from build123d import *

# Parameters (mm, degrees)
SKETCH1_W           = 20
SKETCH1_H           = 405
BOSS_EXTRUDE1_DEPTH = 5
CUT_EXTRUDE1_REACH  = 409.6
SKETCH3_R           = 16.7


with BuildPart() as part:
    # Sketch1 → Revolve1 (revolve)
    with BuildSketch(Plane.XY, mode=Mode.PRIVATE) as revolve1_sk:
        with Locations((10, 202.5)):
            Rectangle(SKETCH1_W, SKETCH1_H)
    revolve(revolve1_sk.sketch.rotate(Axis((0, 405, 0), (0, -1, 0)), 180), axis=Axis((0, 405, 0), (0, -1, 0)))

    # Sketch2 → Boss-Extrude1 (add)
    with BuildSketch(Plane(origin=(0, 405, 0), x_dir=(1, 0, 0), z_dir=(0, 1, 0))):
        with BuildLine():
            Line((-20.5, -32.5), (20.5, -32.5))
            ThreePointArc((20.5, -32.5), (28.985281374, -28.985281374), (32.5, -20.5))
            Line((32.5, -20.5), (32.5, 20.5))
            ThreePointArc((32.5, 20.5), (28.985281374, 28.985281374), (20.5, 32.5))
            Line((20.5, 32.5), (-20.5, 32.5))
            ThreePointArc((-20.5, 32.5), (-28.985281374, 28.985281374), (-32.5, 20.5))
            Line((-32.5, 20.5), (-32.5, -20.5))
            ThreePointArc((-32.5, -20.5), (-28.985281374, -28.985281374), (-20.5, -32.5))
        make_face()
    extrude(amount=-BOSS_EXTRUDE1_DEPTH)

    # Sketch3 → Cut-Extrude1 (cut, up to next)
    with BuildSketch(Plane.XZ, mode=Mode.PRIVATE) as cut_extrude1_sk1:
        Circle(SKETCH3_R)
    cut_extrude1_tool1 = extrude(cut_extrude1_sk1.sketch, amount=-CUT_EXTRUDE1_REACH, mode=Mode.PRIVATE) & part.part
    add(cut_extrude1_tool1.solids().sort_by_distance((0, 0, 0))[0], mode=Mode.SUBTRACT)


solid = part.part
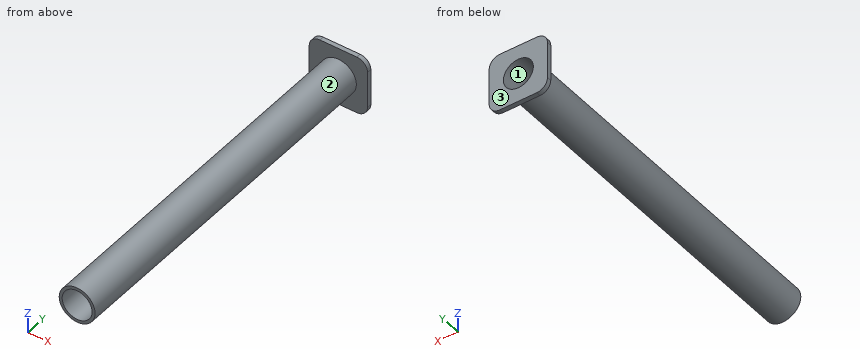
Could you check a few things on this model? Use its own coordinates, in mm. Face numbers are marked on the shaded views. Round coordinates to 2 decimals unless told otherwise and drop trailing zeros. Order: outer loops, then holes, each group sorted by start corner. A loop starts at its lowest first (then second) coordinate and runs counter-clockwise, first axis right, second up.
Q1. Thinking about a two-plate mould opening in Z: for the marked faces 1, 2 and 3, which applies, released by +Z, released by -Z, zero draft, split by the parting line, or undercut?
Geometry says:
face 1: undercut
face 2: split by the parting line
face 3: zero draft
Q2. Imagine slicing it at C-C, the plane y = 134. List the corners of the cut face in (x, z) for me.
Geometry says:
outline: circle Ø40 at (0, 0); hole circle Ø33.4 at (0, 0)
Q3. I'm going to push flat-ended pins straight in: P1, Ø1.5, axis at y = 60, z = 2.5, coming from the -X side; P2, Ø3, axis at x = 15.5, y = 279.5, coming from the -Z side; P3, Ø5, axis at y = 96.5, z = 11, coming from the +X side; P4, Ø20, axis at x = 0, z = 0, coming from the -Y side. Where does each tip first touch, or does it pass through?
Geometry says:
P1: stops at x = -19.92
P2: stops at z = -14.28
P3: stops at x = 18.1
P4: passes through
Q4. Imagine slicing it at A-A, the plane z = 0. List the corners of the cut face in (x, y) for me.
Geometry says:
outline: (-32.5, 400) - (-20, 400) - (-20, 0) - (-16.7, 0) - (-16.7, 405) - (-32.5, 405) - close; (16.7, 0) - (20, 0) - (20, 400) - (32.5, 400) - (32.5, 405) - (16.7, 405) - close
Q5. Imagine slicing it at B-B, the plane x = 0. List the corners of the cut face in (y, z) for me, then the cut area to 3 significant figures.
Geometry says:
outline: (0, -20) - (400, -20) - (400, -32.5) - (405, -32.5) - (405, -16.7) - (0, -16.7) - close; (0, 16.7) - (405, 16.7) - (405, 32.5) - (400, 32.5) - (400, 20) - (0, 20) - close
area: 2,800 mm2
Q6. Please list where these lines run through material, in increasing order: probe 1 along Z at (x, y) = (0, 228); probe 2 along Y at (x, z) = (-10, 26.5); probe 3 along Z at (x, y) = (5.5, 162).
Geometry says:
probe 1: z = -20 to -16.7, 16.7 to 20
probe 2: y = 400 to 405
probe 3: z = -19.23 to -15.77, 15.77 to 19.23
